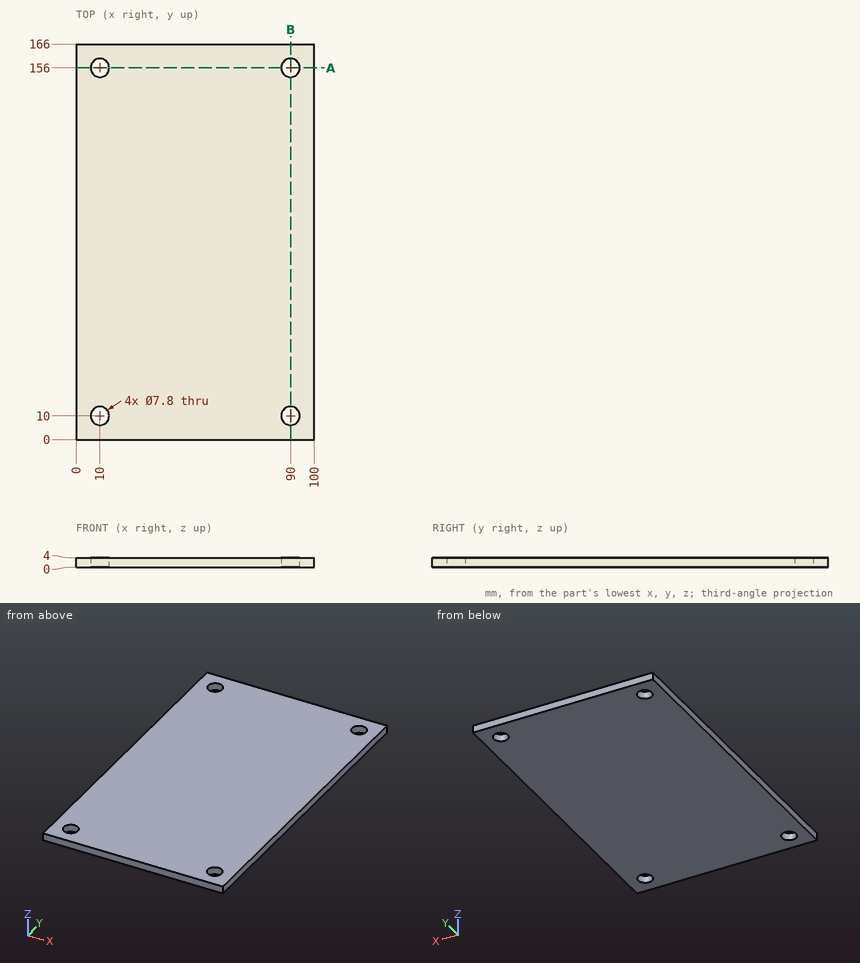
Here's the drawing with two shaded views (mm, measured from the low corner). I have some questions. Give positions to 0.01 mm unless a question says otherwise; leave off trailing zeros. Loops run counter-clockwise (first coordinate to the right, second up) from the corner with the lowest first, then second, coordinate; pieces in that order, holes last. Notation, with made-up numbers: (1, 58) - (54, 58) arc R35 ccw to (54, 90) - close; hole circle Ø6 at (22.25, 5). An arc over 180 degrees is marked (long way). Return JSON: item names as keys, results as strings.
1. I want a section at A-A on y = 156. Please give me the cut outline in (x, z).
Output values:
{"outline": "(0, 0) - (6.1, 0) - (6.1, 4) - (0, 4) - close; (13.9, 0) - (86.1, 0) - (86.1, 4) - (13.9, 4) - close; (93.9, 0) - (100, 0) - (100, 4) - (93.9, 4) - close"}
2. If I drill on line 1 (Y direction, x = 90, z = 2.9); line 2 (X direction, y = 156.5, z = 1.1); line 3 (Y direction, x = 92, z = 2.4), over which ranges is the centre line in solid material (lowest first)?
Output values:
{"line 1": "y = 0 to 6.1, 13.9 to 152.1, 159.9 to 166", "line 2": "x = 0 to 6.13, 13.87 to 86.13, 93.87 to 100", "line 3": "y = 0 to 6.65, 13.35 to 152.65, 159.35 to 166"}
3. I want a section at B-B on x = 90. Please give me the cut outline in (y, z), and give its area (3 significant figures).
Output values:
{"outline": "(0, 0) - (6.1, 0) - (6.1, 4) - (0, 4) - close; (13.9, 0) - (152.1, 0) - (152.1, 4) - (13.9, 4) - close; (159.9, 0) - (166, 0) - (166, 4) - (159.9, 4) - close", "area": "602 mm²"}
4. I'm going to push flat-ended pins straight in: pin 1 Ø12.5 at (x, y) = (90, 10) entering from -Z; pin 2 Ø6 at (x, y) = (90, 156) entering from -Z. Where does each tip first touch, or does it pass through?
Output values:
{"pin 1": "stops at z = 0", "pin 2": "passes through"}
